from build123d import *

# Parameters (mm, degrees)
SKETCH1_W                   = 33
SKETCH1_H                   = 53
SKETCH1_W_2                 = 31
SKETCH1_H_2                 = 51
WALL_HEIGHT_DEPTH           = 18
ROOF_START                  = 18
SKETCH1_3_W                 = 33
SKETCH1_3_H                 = 53
SKETCH1_3_W_2               = 3
SKETCH1_3_H_2               = 3
ROOF_DEPTH                  = 1.5
SKETCH1_5_W                 = 44
SKETCH1_5_H                 = 64
SKETCH1_5_R                 = 1.1303
SKETCH1_5_W_2               = 33
SKETCH1_5_H_2               = 53
SCREW_LIP_DEPTH             = 2
MICRO_D_START               = 18
MICRO_D_FEMALE_CUTOUT_DEPTH = 1.5
FILLET1_R                   = 0.5
SKETCH4_W                   = 44
SKETCH4_H                   = 32
CUT_EXTRUDE3_DEPTH          = 19.5


# Read off the part's stored shape, not the designer's step: Micro-D Female Cutout
with BuildPart() as part:
    # Sketch1 → Wall_Height (new body)
    with BuildSketch(Plane.XY):
        with Locations((16.5, -26.5)):
            Rectangle(SKETCH1_W, SKETCH1_H)
        with Locations((16.5, -26.5)):
            Rectangle(SKETCH1_W_2, SKETCH1_H_2, mode=Mode.SUBTRACT)
    extrude(amount=WALL_HEIGHT_DEPTH)

    # Sketch1<3> → Roof (add)
    with BuildSketch(Plane.XY.offset(ROOF_START)):
        with Locations((16.5, -26.5)):
            Rectangle(SKETCH1_3_W, SKETCH1_3_H)
        with Locations((16.5, -26.5)):
            Rectangle(SKETCH1_3_W_2, SKETCH1_3_H_2, mode=Mode.SUBTRACT)
    extrude(amount=ROOF_DEPTH)

    # Sketch1<5> → Screw_Lip (add)
    with BuildSketch(Plane.XY):
        with Locations((16.5, -26.5)):
            Rectangle(SKETCH1_5_W, SKETCH1_5_H)
        with Locations((35.75, -31.5)):
            Circle(SKETCH1_5_R, mode=Mode.SUBTRACT)
        with Locations((35.75, -21.5)):
            Circle(SKETCH1_5_R, mode=Mode.SUBTRACT)
        with Locations((-2.75, -31.5)):
            Circle(SKETCH1_5_R, mode=Mode.SUBTRACT)
        with Locations((-2.75, -21.5)):
            Circle(SKETCH1_5_R, mode=Mode.SUBTRACT)
        with Locations((35.75, -55.75)):
            Circle(SKETCH1_5_R, mode=Mode.SUBTRACT)
        with Locations((35.75, -26.5)):
            Circle(SKETCH1_5_R, mode=Mode.SUBTRACT)
        with Locations((-2.75, -26.5)):
            Circle(SKETCH1_5_R, mode=Mode.SUBTRACT)
        with Locations((-2.75, -55.75)):
            Circle(SKETCH1_5_R, mode=Mode.SUBTRACT)
        with Locations((-2.75, 2.75)):
            Circle(SKETCH1_5_R, mode=Mode.SUBTRACT)
        with Locations((35.75, 2.75)):
            Circle(SKETCH1_5_R, mode=Mode.SUBTRACT)
        with Locations((16.5, -26.5)):
            Rectangle(SKETCH1_5_W_2, SKETCH1_5_H_2, mode=Mode.SUBTRACT)
    extrude(amount=SCREW_LIP_DEPTH)

    # Micro-D Female Cutout outline → Micro-D Female Cutout (cut)
    with BuildSketch(Plane.XY.offset(MICRO_D_START)):
        with BuildLine():
            Line((9.045291306, -8.922906796), (23.934708694, -8.922906796))
            ThreePointArc((23.934708694, -8.922906796), (25.091998708, -8.574294286), (25.86418098, -7.644463442))
            Line((25.86418098, -7.644463442), (26.936222286, -5.112028361))
            ThreePointArc((26.936222286, -5.112028361), (26.753373348, -3.137945843), (25.00675, -2.2))
            Line((25.00675, -2.2), (7.97325, -2.2))
            ThreePointArc((7.97325, -2.2), (6.226626652, -3.137945843), (6.043777714, -5.112028361))
            Line((6.043777714, -5.112028361), (7.11581902, -7.644463442))
            ThreePointArc((7.11581902, -7.644463442), (7.888001292, -8.574294286), (9.045291306, -8.922906796))
        make_face()
    micro_d_female_cutout = extrude(amount=MICRO_D_FEMALE_CUTOUT_DEPTH, mode=Mode.SUBTRACT)

    # Micro-D Cutout Mirror: Micro-D Female Cutout across plane
    add(micro_d_female_cutout.mirror(Plane.ZX.offset(-26.5)), mode=Mode.SUBTRACT)

    # Fillet1
    fillet1_edges = [part.edges().sort_by_distance(p)[0] for p in [
        (1, -1, 9),
        (1, -52, 9),
        (32, -52, 9),
        (32, -1, 9),
        (15, -28, 18.75),
        (18, -28, 18.75),
        (18, -25, 18.75),
        (15, -25, 18.75),
    ]]
    fillet(fillet1_edges, radius=FILLET1_R)

    # Sketch4 → Cut-Extrude3 (cut)
    with BuildSketch(Plane.XY):
        with Locations((16.5, -42.5)):
            Rectangle(SKETCH4_W, SKETCH4_H)
    extrude(amount=CUT_EXTRUDE3_DEPTH, mode=Mode.SUBTRACT)


solid = part.part
Could you check a few things on this model? Use its own coordinates, in mm. A direction names the side the tool comes from. Coordinates: 2 decimals unless noted, no trailing zeros. Order: outer loops, then holes, each group sorted by start corner. A loop starts at its lowest first (then second) coordinate and runs counter-clockwise, first axis right, second up.
Q1. Suppose I cut it at D-D on z = 11.5. Please give me the cut outline in (x, y).
Q2. Will these pins go through, and if not, where does the flat tip stop? pin 1 (1.5 mm diameter, centred on y = -14.5, z = 13.5, fed in from -X); pin 2 (1.6 mm diameter, centred on x = 18, z = 18.5, fed in from +Y); pin 3 (4 mm diameter, centred on x = 11.5, y = -20, fed in from -Z); pin 4 (1.8 mm diameter, centred on x = -2.75, y = 2.75, fed in from +Z).
Q3. Suppose I cut it at B-B on y = -21.5. Please give me the cut outline in (x, z).
Q4. Suppose I cut it at C-C on x = 35.75. Please give me the cut outline in (y, z).
Q5. Suppose I cut it at A-A on x = 10.5. Please give me the cut outline in (y, z), and give its area (3 significant figures).
Q6. Which directions (+Z, -Z, +X, -X, +Y, -Y) give clear straight access to the entire face, cutting with the end or side of a thin tool? Please do faces 4 (the flat face through (16, -16, 18)), 5 (the cylindrical face through (25.08, -8.58, 18.74)), 6 (the flat face through (18, -26, 19)).
Q7. Please list where these lines run through material, in increasing order: L1, parallel to Y at x = 35.75, z = 1.1; L2, parallel to X at y = -19, z = 6.5; L3, parallel to Y at x = 23.5, z = 18.75.
Q8. Thinking about a two-plate mould opening in X: for faces 1 (the flat face through (16, -13, 19.5)), 2 (the flat face through (17, -2.2, 19)), 3 (the cylindrical face through (36.794, 2.317, 0.986)), which applies, released by +X, released by -X, zero draft, split by the parting line, or undercut?
Answer:
1. outline: (0, -26.5) - (1, -26.5) - (1, -1.5) arc R0.5 cw to (1.5, -1) - (31.5, -1) arc R0.5 cw to (32, -1.5) - (32, -26.5) - (33, -26.5) - (33, 0) - (0, 0) - close
2. pin 1: stops at x = 0
2. pin 2: stops at y = 0
2. pin 3: stops at z = 18
2. pin 4: passes through
3. outline: (-5.5, 0) - (-3.88, 0) - (-3.88, 2) - (-5.5, 2) - close; (-1.62, 0) - (1, 0) - (1, 18) - (32, 18) - (32, 0) - (34.62, 0) - (34.62, 2) - (33, 2) - (33, 19.5) - (0, 19.5) - (0, 2) - (-1.62, 2) - close; (36.88, 0) - (38.5, 0) - (38.5, 2) - (36.88, 2) - close
4. outline: (-25.37, 0) - (-22.63, 0) - (-22.63, 2) - (-25.37, 2) - close; (-20.37, 0) - (1.62, 0) - (1.62, 2) - (-20.37, 2) - close; (3.88, 0) - (5.5, 0) - (5.5, 2) - (3.88, 2) - close
5. outline: (-26.5, 18) - (-8.92, 18) - (-8.92, 19.5) - (-26.5, 19.5) - close; (-2.2, 18) - (-1, 18) - (-1, 0) - (5.5, 0) - (5.5, 2) - (0, 2) - (0, 19.5) - (-2.2, 19.5) - close
5. area: 58.7 mm2
6. face 4: -Z, -Y
6. face 5: +Z, -Z
6. face 6: +Z, -Z, -Y
7. L1: y = -25.37 to -22.63, -20.37 to 1.62, 3.88 to 5.5
7. L2: x = 0 to 1, 32 to 33
7. L3: y = -26.5 to -8.92, -2.2 to 0
8. face 1: zero draft
8. face 2: undercut
8. face 3: undercut
